```python
from build123d import *

# Parameters (mm, degrees)
CYLINDER_R      = 20
CYLINDER_DEPTH  = 3.3
SKETCH_R        = 1.5
POCKET_DEPTH    = 3.301
POCKET001_DEPTH = 3.301


with BuildPart() as part:
    # Cylinder → Cylinder (new body)
    with BuildSketch(Plane.XY):
        Circle(CYLINDER_R)
    extrude(amount=CYLINDER_DEPTH)

    # Sketch → Pocket (cut, through all)
    with BuildSketch(Plane.XY.offset(3.3)):
        with Locations((0, 15.1)):
            Circle(SKETCH_R)
    extrude(amount=-POCKET_DEPTH, mode=Mode.SUBTRACT)

    # Sketch001 → Pocket001 (cut, through all)
    with BuildSketch(Plane(origin=(0, 0, 0), x_dir=(1, 0, 0), z_dir=(0, 0, -1))):
        Polygon((0, 11.547005), (-10, -5.773503), (10, -5.773503), align=None)
    extrude(amount=-POCKET001_DEPTH, mode=Mode.SUBTRACT)


solid = part.part
```
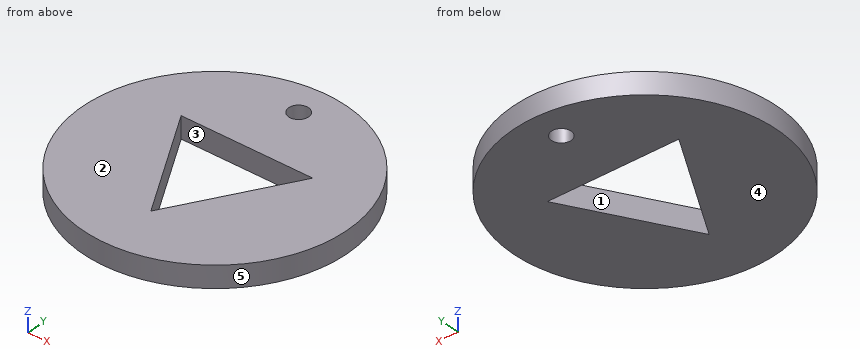
Can you work these out from the model? Positions are in its coordinate system, mm. Face numbers are marked on the shaded views. A direction names the side the tool comes from. Give positions to 0.01 mm unless a question says otherwise; leave off trailing zeros. Order: outer loops, then holes, each group sorted by start corner. A loop starts at its lowest first (then second) coordinate and runs counter-clockwise, first axis right, second up. Notation, with made-up numbers: M 88.5,85.5 L 101.5,85.5 A22 cw 101.5,101.5 Z; hole C -33.5,73 d7. An arc over 180 degrees is marked long. One line per item, written item: value.
1) I want a section at B-B, the plane z = 2.4. List the corners of the cut face in (x, y) for me, plus the area to 3 significant figures.
Answer sheet:
outline: C 0,0 d40; hole M -10,5.77 L 0,-11.55 L 10,5.77 Z; hole C 0,15.1 d3
area: 1,080 mm^2
2) I want a section at A-A, the plane x = 8.5. List the corners of the cut face in (y, z) for me.
Answer sheet:
outline: M -18.1,0 L 3.18,0 L 3.18,3.3 L -18.1,3.3 Z; M 5.77,0 L 18.1,0 L 18.1,3.3 L 5.77,3.3 Z
3) On a 3-axis mill with a long thin cutter (end or side, diameter ignored), from which of +Z, -Z, +X, -X, +Y, -Y can I reach the whole of each face in a straight line? I mean the marked faces 1 and 2. Say none if no direction works.
Answer sheet:
face 1: +Z, -Z
face 2: +Z, +X, -X, +Y, -Y
4) For P1, Ø1, axis at y = 4, z = 0.5, coming from the -X side, with a flat end and sliding along its axis, tell me the tip position at first contact or that it passes through.
Answer sheet:
P1: stops at x = -19.69
5) I want a section at D-D, the plane y = 9.5. List the corners of the cut face in (x, z) for me, plus the area to 3 significant figures.
Answer sheet:
outline: M -17.6,0 L 17.6,0 L 17.6,3.3 L -17.6,3.3 Z
area: 116 mm^2
6) I want a section at C-C, the plane y = 15.1. List the corners of the cut face in (x, z) for me, plus the area to 3 significant figures.
Answer sheet:
outline: M -13.11,0 L -1.5,0 L -1.5,3.3 L -13.11,3.3 Z; M 1.5,0 L 13.11,0 L 13.11,3.3 L 1.5,3.3 Z
area: 76.7 mm^2
7) Please list where these lines run through material, in increasing order: line 1 along Y through (x, z) = (-1, 2.4); line 2 along X through (y, z) = (-10, 2.4); line 3 along Y through (x, z) = (-8, 1.65).
Answer sheet:
line 1: y = -19.97 to -9.81, 5.77 to 13.98, 16.22 to 19.97
line 2: x = -17.32 to -0.89, 0.89 to 17.32
line 3: y = -18.33 to 2.31, 5.77 to 18.33
8) We'd pull the mould along Y, two halves only. Please class the marked faces 3, 4 and 5: released by +Y, released by -Y, zero draft, split by the parting line, or undercut.
Answer sheet:
face 3: undercut
face 4: zero draft
face 5: split by the parting line
